from build123d import *

# Parameters (mm, degrees)
EXTRUDE_1_DEPTH     = 80
FILLET_1_R          = 2
YAW_REACH           = 137.739
SKETCH_2_R          = 2.05
SKETCH_2_R_2        = 9
CUT_EXTRUDE_2_REACH = 135.993
SKETCH_3_R          = 1.55
SKETCH_4_W          = 25
SKETCH_4_H          = 40
CUT_EXTRUDE_3_DEPTH = 171.96490868
FILLET_2_R          = 6
CHAMFER_1_SIZE      = 0.5


with BuildPart() as part:
    # 草图1 → 凸台-拉伸1 (new body)
    with BuildSketch(Plane.XY):
        Polygon((-52, 0), (52, 0), (52, -77), (75, -77), (75, -74), (55, -74), (55, 3), (-55, 3), (-55, -74), (-75, -74), (-75, -77), (-52, -77), align=None)
    extrude(amount=EXTRUDE_1_DEPTH)

    # 圆角1
    fillet_1_edges = [part.edges().sort_by_distance(p)[0] for p in [
        (52, 0, 40),
        (-52, 0, 40),
        (-52, -77, 40),
        (-55, -74, 40),
        (-55, 3, 40),
        (55, 3, 40),
        (55, -74, 40),
        (52, -77, 40),
    ]]
    fillet(fillet_1_edges, radius=FILLET_1_R)

    # 草图2 → yaw (cut, up to next)
    with BuildSketch(Plane(origin=(0, 3, 0), x_dir=(1, 0, 0), z_dir=(0, 1, 0)), mode=Mode.PRIVATE) as yaw_sk1:
        with Locations(Location((-17.320508076, -30, 0), (0, 0, 270))):
            Circle(SKETCH_2_R)
    yaw_tool1 = extrude(yaw_sk1.sketch, amount=-YAW_REACH, mode=Mode.PRIVATE) & part.part
    # 草图2 → yaw (cut, up to next)
    with BuildSketch(Plane(origin=(0, 3, 0), x_dir=(1, 0, 0), z_dir=(0, 1, 0)), mode=Mode.PRIVATE) as yaw_sk2:
        with Locations(Location((0, -20, 0), (0, 0, 270))):
            Circle(SKETCH_2_R)
    yaw_tool2 = extrude(yaw_sk2.sketch, amount=-YAW_REACH, mode=Mode.PRIVATE) & part.part
    # 草图2 → yaw (cut, up to next)
    with BuildSketch(Plane(origin=(0, 3, 0), x_dir=(1, 0, 0), z_dir=(0, 1, 0)), mode=Mode.PRIVATE) as yaw_sk3:
        with Locations(Location((17.320508076, -30, 0), (0, 0, 270))):
            Circle(SKETCH_2_R)
    yaw_tool3 = extrude(yaw_sk3.sketch, amount=-YAW_REACH, mode=Mode.PRIVATE) & part.part
    # 草图2 → yaw (cut, up to next)
    with BuildSketch(Plane(origin=(0, 3, 0), x_dir=(1, 0, 0), z_dir=(0, 1, 0)), mode=Mode.PRIVATE) as yaw_sk4:
        with Locations(Location((17.320508076, -50, 0), (0, 0, 270))):
            Circle(SKETCH_2_R)
    yaw_tool4 = extrude(yaw_sk4.sketch, amount=-YAW_REACH, mode=Mode.PRIVATE) & part.part
    # 草图2 → yaw (cut, up to next)
    with BuildSketch(Plane(origin=(0, 3, 0), x_dir=(1, 0, 0), z_dir=(0, 1, 0)), mode=Mode.PRIVATE) as yaw_sk5:
        with Locations(Location((0, -40, 0), (0, 0, 270))):
            Circle(SKETCH_2_R_2)
    yaw_tool5 = extrude(yaw_sk5.sketch, amount=-YAW_REACH, mode=Mode.PRIVATE) & part.part
    # 草图2 → yaw (cut, up to next)
    with BuildSketch(Plane(origin=(0, 3, 0), x_dir=(1, 0, 0), z_dir=(0, 1, 0)), mode=Mode.PRIVATE) as yaw_sk6:
        with Locations(Location((0, -60, 0), (0, 0, 270))):
            Circle(SKETCH_2_R)
    yaw_tool6 = extrude(yaw_sk6.sketch, amount=-YAW_REACH, mode=Mode.PRIVATE) & part.part
    # 草图2 → yaw (cut, up to next)
    with BuildSketch(Plane(origin=(0, 3, 0), x_dir=(1, 0, 0), z_dir=(0, 1, 0)), mode=Mode.PRIVATE) as yaw_sk7:
        with Locations(Location((-17.320508076, -50, 0), (0, 0, 270))):
            Circle(SKETCH_2_R)
    yaw_tool7 = extrude(yaw_sk7.sketch, amount=-YAW_REACH, mode=Mode.PRIVATE) & part.part
    add(yaw_tool1.solids().sort_by_distance((-17.320508, 3, 30))[0], mode=Mode.SUBTRACT)
    add(yaw_tool2.solids().sort_by_distance((0, 3, 20))[0], mode=Mode.SUBTRACT)
    add(yaw_tool3.solids().sort_by_distance((17.320508, 3, 30))[0], mode=Mode.SUBTRACT)
    add(yaw_tool4.solids().sort_by_distance((17.320508, 3, 50))[0], mode=Mode.SUBTRACT)
    add(yaw_tool5.solids().sort_by_distance((0, 3, 40))[0], mode=Mode.SUBTRACT)
    add(yaw_tool6.solids().sort_by_distance((0, 3, 60))[0], mode=Mode.SUBTRACT)
    add(yaw_tool7.solids().sort_by_distance((-17.320508, 3, 50))[0], mode=Mode.SUBTRACT)

    # 草图3 → 切除-拉伸2 (cut, up to next)
    with BuildSketch(Plane(origin=(0, -74, 0), x_dir=(1, 0, 0), z_dir=(0, 1, 0)), mode=Mode.PRIVATE) as cut_extrude_2_sk1:
        with Locations(Location((-66, -10, 0), (0, 0, 270))):
            Circle(SKETCH_3_R)
    cut_extrude_2_tool1 = extrude(cut_extrude_2_sk1.sketch, amount=-CUT_EXTRUDE_2_REACH, mode=Mode.PRIVATE) & part.part
    # 草图3 → 切除-拉伸2 (cut, up to next)
    with BuildSketch(Plane(origin=(0, -74, 0), x_dir=(1, 0, 0), z_dir=(0, 1, 0)), mode=Mode.PRIVATE) as cut_extrude_2_sk2:
        with Locations(Location((-66, -30, 0), (0, 0, 270))):
            Circle(SKETCH_3_R)
    cut_extrude_2_tool2 = extrude(cut_extrude_2_sk2.sketch, amount=-CUT_EXTRUDE_2_REACH, mode=Mode.PRIVATE) & part.part
    # 草图3 → 切除-拉伸2 (cut, up to next)
    with BuildSketch(Plane(origin=(0, -74, 0), x_dir=(1, 0, 0), z_dir=(0, 1, 0)), mode=Mode.PRIVATE) as cut_extrude_2_sk3:
        with Locations(Location((-66, -50, 0), (0, 0, 270))):
            Circle(SKETCH_3_R)
    cut_extrude_2_tool3 = extrude(cut_extrude_2_sk3.sketch, amount=-CUT_EXTRUDE_2_REACH, mode=Mode.PRIVATE) & part.part
    # 草图3 → 切除-拉伸2 (cut, up to next)
    with BuildSketch(Plane(origin=(0, -74, 0), x_dir=(1, 0, 0), z_dir=(0, 1, 0)), mode=Mode.PRIVATE) as cut_extrude_2_sk4:
        with Locations(Location((-66, -70, 0), (0, 0, 270))):
            Circle(SKETCH_3_R)
    cut_extrude_2_tool4 = extrude(cut_extrude_2_sk4.sketch, amount=-CUT_EXTRUDE_2_REACH, mode=Mode.PRIVATE) & part.part
    # 草图3 → 切除-拉伸2 (cut, up to next)
    with BuildSketch(Plane(origin=(0, -74, 0), x_dir=(1, 0, 0), z_dir=(0, 1, 0)), mode=Mode.PRIVATE) as cut_extrude_2_sk5:
        with Locations(Location((66, -70, 0), (0, 0, 270))):
            Circle(SKETCH_3_R)
    cut_extrude_2_tool5 = extrude(cut_extrude_2_sk5.sketch, amount=-CUT_EXTRUDE_2_REACH, mode=Mode.PRIVATE) & part.part
    # 草图3 → 切除-拉伸2 (cut, up to next)
    with BuildSketch(Plane(origin=(0, -74, 0), x_dir=(1, 0, 0), z_dir=(0, 1, 0)), mode=Mode.PRIVATE) as cut_extrude_2_sk6:
        with Locations(Location((66, -50, 0), (0, 0, 270))):
            Circle(SKETCH_3_R)
    cut_extrude_2_tool6 = extrude(cut_extrude_2_sk6.sketch, amount=-CUT_EXTRUDE_2_REACH, mode=Mode.PRIVATE) & part.part
    # 草图3 → 切除-拉伸2 (cut, up to next)
    with BuildSketch(Plane(origin=(0, -74, 0), x_dir=(1, 0, 0), z_dir=(0, 1, 0)), mode=Mode.PRIVATE) as cut_extrude_2_sk7:
        with Locations(Location((66, -30, 0), (0, 0, 270))):
            Circle(SKETCH_3_R)
    cut_extrude_2_tool7 = extrude(cut_extrude_2_sk7.sketch, amount=-CUT_EXTRUDE_2_REACH, mode=Mode.PRIVATE) & part.part
    # 草图3 → 切除-拉伸2 (cut, up to next)
    with BuildSketch(Plane(origin=(0, -74, 0), x_dir=(1, 0, 0), z_dir=(0, 1, 0)), mode=Mode.PRIVATE) as cut_extrude_2_sk8:
        with Locations(Location((66, -10, 0), (0, 0, 270))):
            Circle(SKETCH_3_R)
    cut_extrude_2_tool8 = extrude(cut_extrude_2_sk8.sketch, amount=-CUT_EXTRUDE_2_REACH, mode=Mode.PRIVATE) & part.part
    add(cut_extrude_2_tool1.solids().sort_by_distance((-66, -74, 10))[0], mode=Mode.SUBTRACT)
    add(cut_extrude_2_tool2.solids().sort_by_distance((-66, -74, 30))[0], mode=Mode.SUBTRACT)
    add(cut_extrude_2_tool3.solids().sort_by_distance((-66, -74, 50))[0], mode=Mode.SUBTRACT)
    add(cut_extrude_2_tool4.solids().sort_by_distance((-66, -74, 70))[0], mode=Mode.SUBTRACT)
    add(cut_extrude_2_tool5.solids().sort_by_distance((66, -74, 70))[0], mode=Mode.SUBTRACT)
    add(cut_extrude_2_tool6.solids().sort_by_distance((66, -74, 50))[0], mode=Mode.SUBTRACT)
    add(cut_extrude_2_tool7.solids().sort_by_distance((66, -74, 30))[0], mode=Mode.SUBTRACT)
    add(cut_extrude_2_tool8.solids().sort_by_distance((66, -74, 10))[0], mode=Mode.SUBTRACT)

    # 草图4 → 切除-拉伸3 (cut, through all)
    with BuildSketch(Plane.ZY.offset(55)):
        with Locations((40, -39)):
            Rectangle(SKETCH_4_W, SKETCH_4_H)
    extrude(amount=-CUT_EXTRUDE_3_DEPTH, mode=Mode.SUBTRACT)

    # 圆角2
    fillet_2_edges = [part.edges().sort_by_distance(p)[0] for p in [
        (53.5, -19, 52.5),
        (-53.5, -19, 52.5),
        (53.5, -59, 52.5),
        (-53.5, -59, 52.5),
        (53.5, -59, 27.5),
        (-53.5, -59, 27.5),
        (53.5, -19, 27.5),
        (-53.5, -19, 27.5),
    ]]
    fillet(fillet_2_edges, radius=FILLET_2_R)

    # 倒角1
    chamfer_1_edges = [part.edges().sort_by_distance(p)[0] for p in [
        (-64.5, -77, 0),
        (66, -74, 80),
        (66, -74, 0),
        (55, -39, 27.5),
        (52, -39, 27.5),
        (55, -19, 40),
        (52, -19, 40),
        (55, -39, 52.5),
        (52, -39, 52.5),
        (55, -59, 40),
        (52, -59, 40),
        (-55, -59, 40),
        (-52, -59, 40),
        (-55, -39, 27.5),
        (-52, -39, 27.5),
        (-55, -39, 52.5),
        (-52, -39, 52.5),
        (-55, -19, 40),
        (-52, -19, 40),
        (52, -20.757359313, 29.257359313),
        (55, -20.757359313, 29.257359313),
        (52, -20.757359313, 50.742640687),
        (55, -20.757359313, 50.742640687),
        (52, -57.242640687, 50.742640687),
        (55, -57.242640687, 50.742640687),
        (52, -57.242640687, 29.257359313),
        (55, -57.242640687, 29.257359313),
        (-55, -57.242640687, 29.257359313),
        (-52, -57.242640687, 29.257359313),
        (-55, -57.242640687, 50.742640687),
        (-75, -77, 40),
        (-52, -57.242640687, 50.742640687),
        (-55, -20.757359313, 50.742640687),
        (-52, -20.757359313, 50.742640687),
        (-75, -74, 40),
        (-55, -20.757359313, 29.257359313),
        (-52, -20.757359313, 29.257359313),
        (75, -74, 40),
        (75, -77, 40),
        (-64.5, -77, 80),
        (0, 3, 0),
        (0, 3, 80),
        (52, -38.5, 0),
        (0, 0, 0),
        (-52, -38.5, 0),
        (-66, -74, 0),
        (-55, -35.5, 0),
        (55, -35.5, 0),
        (64.5, -77, 0),
        (-52.585786438, -76.414213562, 0),
        (52.585786438, -76.414213562, 0),
        (-54.414213562, 2.414213562, 0),
        (54.414213562, 2.414213562, 0),
        (55, -35.5, 80),
        (52, -38.5, 80),
        (64.5, -77, 80),
        (-55, -35.5, 80),
        (-66, -74, 80),
        (-52, -38.5, 80),
        (0, 0, 80),
        (-52.585786438, -76.414213562, 80),
        (52.585786438, -76.414213562, 80),
        (-54.414213562, 2.414213562, 80),
        (54.414213562, 2.414213562, 80),
        (-51.414213562, -0.585786438, 0),
        (-51.414213562, -0.585786438, 80),
        (51.414213562, -0.585786438, 0),
        (51.414213562, -0.585786438, 80),
        (55.585786438, -73.414213562, 0),
        (55.585786438, -73.414213562, 80),
        (-55.585786438, -73.414213562, 0),
        (-55.585786438, -73.414213562, 80),
    ]]
    chamfer(chamfer_1_edges, length=CHAMFER_1_SIZE)


solid = part.part
Geometry check sheet. Reference: the model listing, model coordinates, mm. A direction names the side the tool comes from. Give positions to 0.01 mm unless a question says otherwise; leave off trailing zeros. Loops run counter-clockwise (first coordinate to the right, second up) from the corner with the lowest first, then second, coordinate; pieces in that order, holes last. Notation, with made-up numbers: M 66,71 L 73,71 A35 cw 73,104 Z; hole C 63,73.25 d7. An arc over 180 degrees is marked long. Answer as a JSON object with one key per item and string values. Group by question number.
Item 1: Sectioned sample at D-D on z = 60. Record the boundary of the cut face in (x, y).
Item 2: Material ranges on L1, parallel to Z at x = -66, y = -75.95; L2, parallel to X at y = -47, z = 59; L3, parallel to X at y = -75, z = 30, recorded low to high.
Item 3: Mould release check, pull along Z, two halves, no side actions. Record for faces 1 (the cylindrical face through (-53.486, -57.289, 50.696)), 2 (the flat face through (66, -74, 39)): pulls with the +Z half, pulls with the -Z half, needs draft (parallel to the pull), parting line crosses it, or undercut.
Item 4: Access from +Z, -Z, +X, -X, +Y, -Y to the whole of each face (thin tool, end or side, straight path). Record for faces 3 (the conical face through (52.36, -57.29, 29.11)), 4 (the conical face through (54.64, -57.29, 50.89)), 5 (the conical face through (-54.642, -57.391, 50.795)), 6 (the flat face through (55, -36, 22)), 7 (the cylindrical face through (-53.486, -20.711, 29.304)).
Item 5: Gauge pin test, flat ends, axial feed: pin 1 (1.6 mm diameter, centred on x = 54, z = 37, fed in from +Y); pin 2 (1.6 mm diameter, centred on x = 53, z = 40.5, fed in from -Y); pin 3 (12 mm diameter, centred on y = -15, z = 36.5, fed in from -X). Record the tip position at first contact, or that the pin passes through.
Item 6: Sectioned sample at C-C on x = -66. Record the boundary of the cut face in (y, z).
Item 7: Sectioned sample at A-A on z = 10. Give the number of separate pieces and of enclosed holes in the cut face, plus the area to 3 significant figures.
Findings below:
{
 "1": {"outline": "M -75,-76.5 L -74.5,-77 L -54,-77 A2 ccw -52,-75 L -52,-2 A2 cw -50,0 L -2.05,0 L -2.05,3 L -53,3 A2 ccw -55,1 L -55,-72 A2 cw -57,-74 L -74.5,-74 L -75,-74.5 Z; M 2.05,0 L 50,0 A2 cw 52,-2 L 52,-75 A2 ccw 54,-77 L 74.5,-77 L 75,-76.5 L 75,-74.5 L 74.5,-74 L 57,-74 A2 cw 55,-72 L 55,1 A2 ccw 53,3 L 2.05,3 Z"},
 "2": {"L1": "0 to 8.45, 11.55 to 28.45, 31.55 to 48.45, 51.55 to 68.45, 71.55 to 80", "L2": "-55 to -52, 52 to 55", "L3": "-75 to -67.55, -64.45 to -52, 52 to 64.45, 67.55 to 75"},
 "3": {"face 1": "undercut", "face 2": "needs draft"},
 "4": {"face 3": "none", "face 4": "+X", "face 5": "-X", "face 6": "+Z, -Z, +X, +Y", "face 7": "+X, -X"},
 "5": {"pin 1": "y = 2.99", "pin 2": "y = -76.99", "pin 3": "x = -55"},
 "6": {"outline": "M -77,0.5 L -76.5,0 L -74.5,0 L -74,0.5 L -74,8.45 L -77,8.45 Z; M -77,11.55 L -74,11.55 L -74,28.45 L -77,28.45 Z; M -77,31.55 L -74,31.55 L -74,48.45 L -77,48.45 Z; M -77,51.55 L -74,51.55 L -74,68.45 L -77,68.45 Z; M -77,71.55 L -74,71.55 L -74,79.5 L -74.5,80 L -76.5,80 L -77,79.5 Z"},
 "7": {"separate pieces": "3", "enclosed holes": "0", "area": "893 mm2"}
}
